Here's how the part is built. I have some questions about the finished solid (model axes, mm). Round coordinates to 2 decimals unless told otherwise and drop trailing zeros. Write each loop counter-clockwise with the first axis right and the second up, starting at its lowest first coordinate (ties: lowest second). Pieces come first, ordered by that corner, then holes. Notation, with made-up numbers: (47.5, 74) -> (59.5, 74) arc R23 ccw to (59.5, 86) -> close; hole circle Ø6 at (-31, -28). An arc over 180 degrees is marked (long way). Answer in a Markdown table with one row per item.
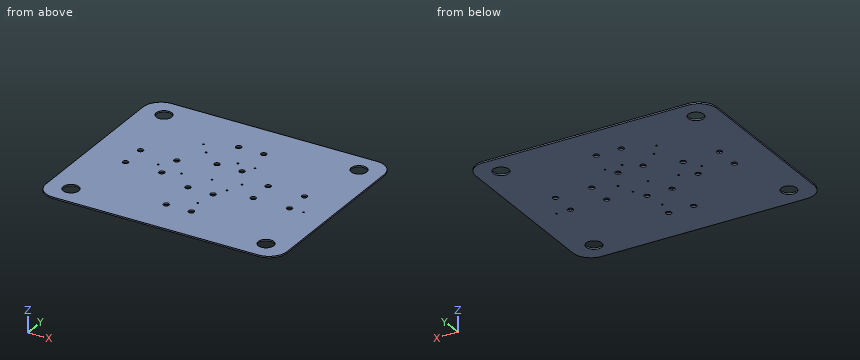
from build123d import *

# Parameters (mm, degrees)
BOARD_OUTLINE_START = 0.034
BOARD_OUTLINE_DEPTH = 0.254
SKETCH2_R           = 1.397
NPTH_DEPTH          = 1.288
SKETCH3_R           = 0.5
SKETCH3_R_2         = 0.1525
PTH_DEPTH           = 1.288


with BuildPart() as part:
    # Sketch1 → Board_Outline (new body)
    with BuildSketch(Plane.XY.offset(BOARD_OUTLINE_START)):
        with BuildLine():
            Line((-21.565, 14.63), (-21.565, -14.63))
            ThreePointArc((-21.565, -14.63), (-20.655306988, -16.845306988), (-18.44, -17.755))
            Line((-18.44, -17.755), (18.364, -17.755))
            ThreePointArc((18.364, -17.755), (20.620097217, -16.810097217), (21.565, -14.554))
            Line((21.565, -14.554), (21.565, 14.63))
            ThreePointArc((21.565, 14.63), (20.651306754, 16.841306754), (18.44, 17.755))
            Line((18.44, 17.755), (-18.364, 17.755))
            ThreePointArc((-18.364, 17.755), (-20.588664714, 16.8318444), (-21.565, 14.63))
        make_face()
    extrude(amount=BOARD_OUTLINE_DEPTH)

    # Sketch2 → NPTH (cut, through all)
    with BuildSketch(Plane.XY):
        with Locations((-17.462, 13.97)):
            Circle(SKETCH2_R)
        with Locations((17.462, -13.97)):
            Circle(SKETCH2_R)
        with Locations((17.462, 13.97)):
            Circle(SKETCH2_R)
        with Locations((-17.462, -13.97)):
            Circle(SKETCH2_R)
    extrude(amount=NPTH_DEPTH, mode=Mode.SUBTRACT)

    # Sketch3 → PTH (cut, through all)
    with BuildSketch(Plane.XY):
        with Locations((-2.25, 10.87)):
            Circle(SKETCH3_R)
        with Locations((2.25, 10.87)):
            Circle(SKETCH3_R)
        with Locations((2.25, 4.37)):
            Circle(SKETCH3_R)
        with Locations((-2.25, 4.37)):
            Circle(SKETCH3_R)
        with Locations((-8.18, 2.25)):
            Circle(SKETCH3_R)
        with Locations((-8.18, -2.25)):
            Circle(SKETCH3_R)
        with Locations((-14.68, -2.25)):
            Circle(SKETCH3_R)
        with Locations((-14.68, 2.25)):
            Circle(SKETCH3_R)
        with Locations((-2.25, -4.37)):
            Circle(SKETCH3_R)
        with Locations((2.25, -4.37)):
            Circle(SKETCH3_R)
        with Locations((2.25, -10.87)):
            Circle(SKETCH3_R)
        with Locations((-2.25, -10.87)):
            Circle(SKETCH3_R)
        with Locations((14.68, 2.25)):
            Circle(SKETCH3_R)
        with Locations((14.68, -2.25)):
            Circle(SKETCH3_R)
        with Locations((8.18, -2.25)):
            Circle(SKETCH3_R)
        with Locations((8.18, 2.25)):
            Circle(SKETCH3_R)
        with Locations((4.45, 0.635)):
            Circle(SKETCH3_R_2)
        with Locations((-7.366, 8.89)):
            Circle(SKETCH3_R_2)
        with Locations((3.43, -2.148)):
            Circle(SKETCH3_R_2)
        with Locations((3.43, 6.223)):
            Circle(SKETCH3_R_2)
        with Locations((-9.944, -0.354)):
            Circle(SKETCH3_R_2)
        with Locations((-0.313, -0.354)):
            Circle(SKETCH3_R_2)
        with Locations((0.398, 6.223)):
            Circle(SKETCH3_R_2)
        with Locations((-5.377, -1.065)):
            Circle(SKETCH3_R_2)
        with Locations((17.196, -2.25)):
            Circle(SKETCH3_R_2)
        with Locations((1.666, -8.001)):
            Circle(SKETCH3_R_2)
        with Locations((-5.645, 6.807)):
            Circle(SKETCH3_R_2)
    extrude(amount=PTH_DEPTH, mode=Mode.SUBTRACT)


solid = part.part
1) For pin 1 (2 mm diameter, centred on x = -17.462, y = 13.97, fed in from +Z), with a flat end and sliding along its axis, tell me the tip position at first contact or that it passes through.
Response:
| item | result |
|---|---|
| pin 1 | passes through |
2) I need wall thicknesses on line 1 (X direction, y = -4.37, z = 0.25) (3 decimals); line 2 (Y direction, x = 8.18, z = 0.15) (3 decimals); line 3 (X direction, y = 13.97, z = 0.25) (3 decimals). Which ranges of each line are inside material? Lowest first, please. Write a range as [from, to].
Response:
| item | result |
|---|---|
| line 1 | x = [-21.565, -2.75], [-1.75, 1.75], [2.75, 21.565] |
| line 2 | y = [-17.755, -2.75], [-1.75, 1.75], [2.75, 17.755] |
| line 3 | x = [-21.565, -18.859], [-16.065, 16.065], [18.859, 21.565] |
3) I want a section at D-D, the plane z = 0.2. Count the separate pieces of the cut face and the enclosed holes in it, and give its area (3 significant figures).
Response:
| item | result |
|---|---|
| separate pieces | 1 |
| enclosed holes | 31 |
| area | 1,490 mm^2 |
4) I want a section at A-A, the plane x = -8.18. List the corners of the cut face in (y, z) for me (3 decimals), and give its area (3 significant figures).
Response:
| item | result |
|---|---|
| outline | (-17.755, 0.034) -> (-2.75, 0.034) -> (-2.75, 0.288) -> (-17.755, 0.288) -> close; (-1.75, 0.034) -> (1.75, 0.034) -> (1.75, 0.288) -> (-1.75, 0.288) -> close; (2.75, 0.034) -> (17.755, 0.034) -> (17.755, 0.288) -> (2.75, 0.288) -> close |
| area | 8.51 mm^2 |
5) I want a section at B-B, the plane y = -10.87. List the corners of the cut face in (x, z) for me (3 decimals).
Response:
| item | result |
|---|---|
| outline | (-21.565, 0.034) -> (-2.75, 0.034) -> (-2.75, 0.288) -> (-21.565, 0.288) -> close; (-1.75, 0.034) -> (1.75, 0.034) -> (1.75, 0.288) -> (-1.75, 0.288) -> close; (2.75, 0.034) -> (21.565, 0.034) -> (21.565, 0.288) -> (2.75, 0.288) -> close |
6) I want a section at C-C, the plane x = -2.25. List the corners of the cut face in (y, z) for me (3 decimals).
Response:
| item | result |
|---|---|
| outline | (-17.755, 0.034) -> (-11.37, 0.034) -> (-11.37, 0.288) -> (-17.755, 0.288) -> close; (-10.37, 0.034) -> (-4.87, 0.034) -> (-4.87, 0.288) -> (-10.37, 0.288) -> close; (-3.87, 0.034) -> (3.87, 0.034) -> (3.87, 0.288) -> (-3.87, 0.288) -> close; (4.87, 0.034) -> (10.37, 0.034) -> (10.37, 0.288) -> (4.87, 0.288) -> close; (11.37, 0.034) -> (17.755, 0.034) -> (17.755, 0.288) -> (11.37, 0.288) -> close |
